Could you check a few things on this drawing? It's one solid part, dimensions in mm from its lowest x, y, z. A direction names the side the tool comes from. Give positions to 0.01 mm unless a question says otherwise; leave off trailing zeros. Order: outer loops, then holes, each group sorted by start corner. A loop starts at its lowest first (then second) coordinate and runs counter-clockwise, first axis right, second up.
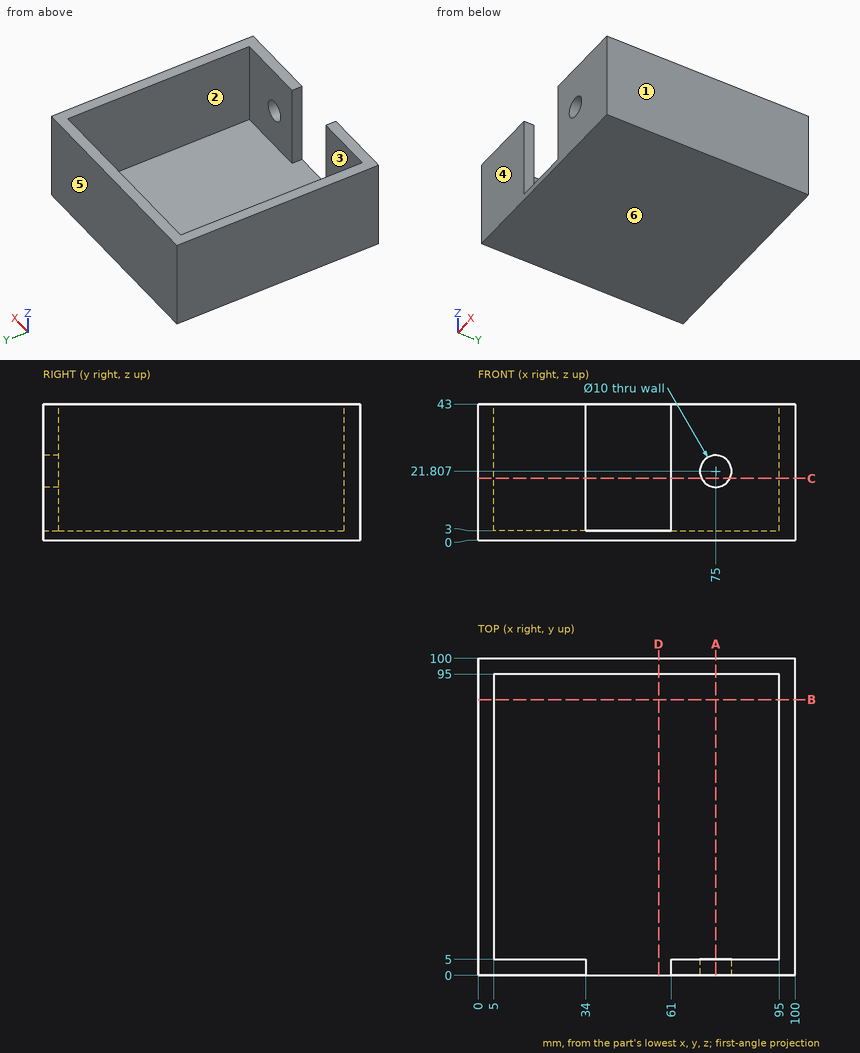
1) If I drill on line 1 (Y direction, x = 69.5, z = 20); line 2 (Z direction, x = 75, y = 1.9), over which ranges is the centre line in solid material (lowest first)?
2) Which directions (+Z, -Z, +X, -X, +Y, -Y) give clear straight access to the entire face, cutting with the end or side of a thin tool? Please do the marked faces 1 and 2.
3) We'd pull the mould along Y, two halves only. Please class the marked faces 3, 4, 5 and 6: +Y half, -Y half, draft (parallel to the pull), parting line (faces both ways), or undercut.
4) Suppose I cut it at C-C (z = 19.5). Please give me the cut outline in (x, y).
5) Suppose I cut it at D-D (x = 57). Please give me the cut outline in (y, z).
6) I'm going to push flat-ended pins straight in: pin 1 Ø12 at (x, y) = (63, 74.5) entering from +Z; pin 2 Ø9 at (x, z) = (75, 21.81) entering from -Y. Where does each tip first touch, or does it pass through?
7) Suppose I cut it at B-B (y = 87). Please give me the cut outline in (x, z).
8) Suppose I cut it at A-A (x = 75). Please give me the cut outline in (y, z).
Results:
1. line 1: y = 0 to 5, 95 to 100
1. line 2: z = 0 to 16.81, 26.81 to 43
2. face 1: +Z, -Z, +X, +Y, -Y
2. face 2: +Z
3. face 3: undercut
3. face 4: -Y half
3. face 5: +Y half
3. face 6: draft
4. outline: (0, 0) - (34, 0) - (34, 5) - (5, 5) - (5, 95) - (95, 95) - (95, 5) - (79.44, 5) - (79.44, 0) - (100, 0) - (100, 100) - (0, 100) - close; (61, 0) - (70.56, 0) - (70.56, 5) - (61, 5) - close
5. outline: (0, 0) - (100, 0) - (100, 43) - (95, 43) - (95, 3) - (0, 3) - close
6. pin 1: stops at z = 3
6. pin 2: stops at y = 95
7. outline: (0, 0) - (100, 0) - (100, 43) - (95, 43) - (95, 3) - (5, 3) - (5, 43) - (0, 43) - close
8. outline: (0, 0) - (100, 0) - (100, 43) - (95, 43) - (95, 3) - (5, 3) - (5, 16.81) - (0, 16.81) - close; (0, 26.81) - (5, 26.81) - (5, 43) - (0, 43) - close
